from build123d import *

# Parameters (mm, degrees)
BOX168_W                  = 6
BOX168_H                  = 121
BOX168_DEPTH              = 172
BOX169_W                  = 40
BOX169_H                  = 100
BOX169_DEPTH              = 135
FUSION057_ROLL_ANGLE      = -90
FUSION057_PLACEMENT_ANGLE = 90


with BuildPart() as cube128:
    # Box168 → Box168 (new body)
    with BuildSketch(Plane.XY):
        with Locations((3, 60.5)):
            Rectangle(BOX168_W, BOX168_H)
    extrude(amount=BOX168_DEPTH)


with BuildPart() as f_120_roll_holder:
    # Box169 → Box169 (new body)
    with BuildSketch(Plane(origin=(-39, 13, 7), x_dir=(1, 0, 0), z_dir=(0, 0, 1))):
        with Locations((20, 50)):
            Rectangle(BOX169_W, BOX169_H)
    extrude(amount=BOX169_DEPTH)

    # Fusion057: union Cube128
    add(cube128.part)


with BuildPart() as f_120_roll_holder_1:
    # Fusion057 roll: moved
    add(f_120_roll_holder.part.rotate(Axis((0, 0, 0), (1, 0, 0)), FUSION057_ROLL_ANGLE))


with BuildPart() as f_120_roll_holder_2:
    # Fusion057 placement: moved
    add(f_120_roll_holder_1.part.moved(Location((162, 0.5, 175))).rotate(Axis((162, 0.5, 175), (0, 0, 1)), FUSION057_PLACEMENT_ANGLE))


solid = f_120_roll_holder_2.part
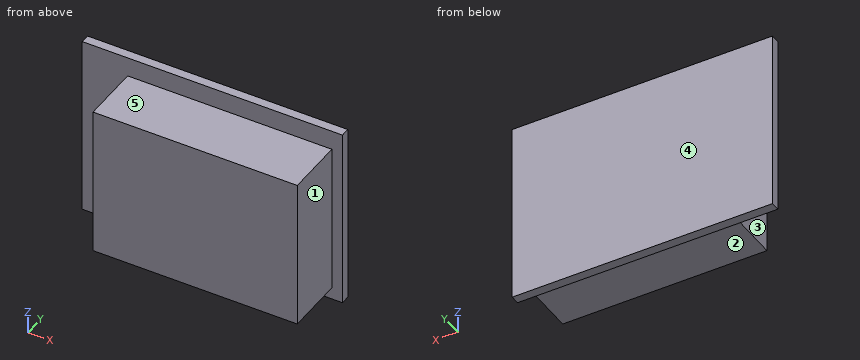
Read the model definition and answer for the solid it produces. Units are mm, in the model's axes. Face numbers are marked on the shaded views. A direction names the side the tool comes from. Coordinates: 2 decimals unless noted, no trailing zeros. Loops run counter-clockwise (first coordinate to the right, second up) from the corner with the lowest first, then second, coordinate; pieces in that order, holes last. Notation, with made-up numbers: (-25, 18) -> (5, 18) arc R15 cw to (5, 34) -> close; hole circle Ø6 at (15.25, 9.5). An arc over 180 degrees is marked (long way). Answer in a Markdown table with one row per item.
Item 1: For the marked faces 1, 2, 3, 4 and 5, determine the directions among +Z, -Z, +X, -X, +Y, -Y from which every point of the face is accessible in a straight line to the end or side of a thin tool.
Returned:
| item | result |
|---|---|
| face 1 | +Z, -Z, +X, -Y |
| face 2 | -Z, +X, -X, -Y |
| face 3 | +Z, -Z, -X, -Y |
| face 4 | +Z, -Z, +X, -X, +Y |
| face 5 | +Z, +X, -X, -Y |
Item 2: Each of these flat-tipped pins is pushed along its axis until it touches: P1, Ø4, axis at x = 106, y = -15, coming from the +Z side; P2, Ø2, axis at x = 95.5, y = -8, coming from the -Z side; P3, Ø12, axis at y = -31, z = 119, coming from the +X side. Where does it stop, or does it pass through?
Returned:
| item | result |
|---|---|
| P1 | stops at z = 162 |
| P2 | stops at z = 62 |
| P3 | stops at x = 155 |
Item 3: A cutting plane is placed at B-B on x = 80.5. Determine the outline of the cut face in (y, z).
Returned:
| item | result |
|---|---|
| outline | (-38.5, 62) -> (0.5, 62) -> (0.5, 54) -> (6.5, 54) -> (6.5, 175) -> (0.5, 175) -> (0.5, 162) -> (-38.5, 162) -> close |
Item 4: A cutting plane is placed at A-A on z = 109. Determine the outline of the cut face in (x, y).
Returned:
| item | result |
|---|---|
| outline | (-10, 0.5) -> (20, 0.5) -> (20, -38.5) -> (155, -38.5) -> (155, 0.5) -> (162, 0.5) -> (162, 6.5) -> (-10, 6.5) -> close |
Item 5: A cutting plane is placed at C-C on y = -24. Determine the outline of the cut face in (x, z).
Returned:
| item | result |
|---|---|
| outline | (20, 62) -> (155, 62) -> (155, 162) -> (20, 162) -> close |
Item 6: A cutting plane is placed at D-D on x = 10. Determine the outline of the cut face in (y, z).
Returned:
| item | result |
|---|---|
| outline | (0.5, 54) -> (6.5, 54) -> (6.5, 175) -> (0.5, 175) -> close |
Item 7: Straight lines are drawn through the part: line 1 along X through (y, z) = (-21, 78); line 2 along Z through (x, y) = (136.5, -30.5); line 3 along Y through (x, z) = (137, 164). For each, find the intervals that lie inside material, in ascending order. Write a range as [from, to].
Returned:
| item | result |
|---|---|
| line 1 | x = [20, 155] |
| line 2 | z = [62, 162] |
| line 3 | y = [0.5, 6.5] |
